Geometry check sheet. Reference: drawing and pictorial views, mm from the part's lowest x, y, z. A direction names the side the tool comes from. Give positions to 0.01 mm unless a question says otherwise; leave off trailing zeros. Order: outer loops, then holes, each group sorted by start corner. A loop starts at its lowest first (then second) coordinate and runs counter-clockwise, first axis right, second up.
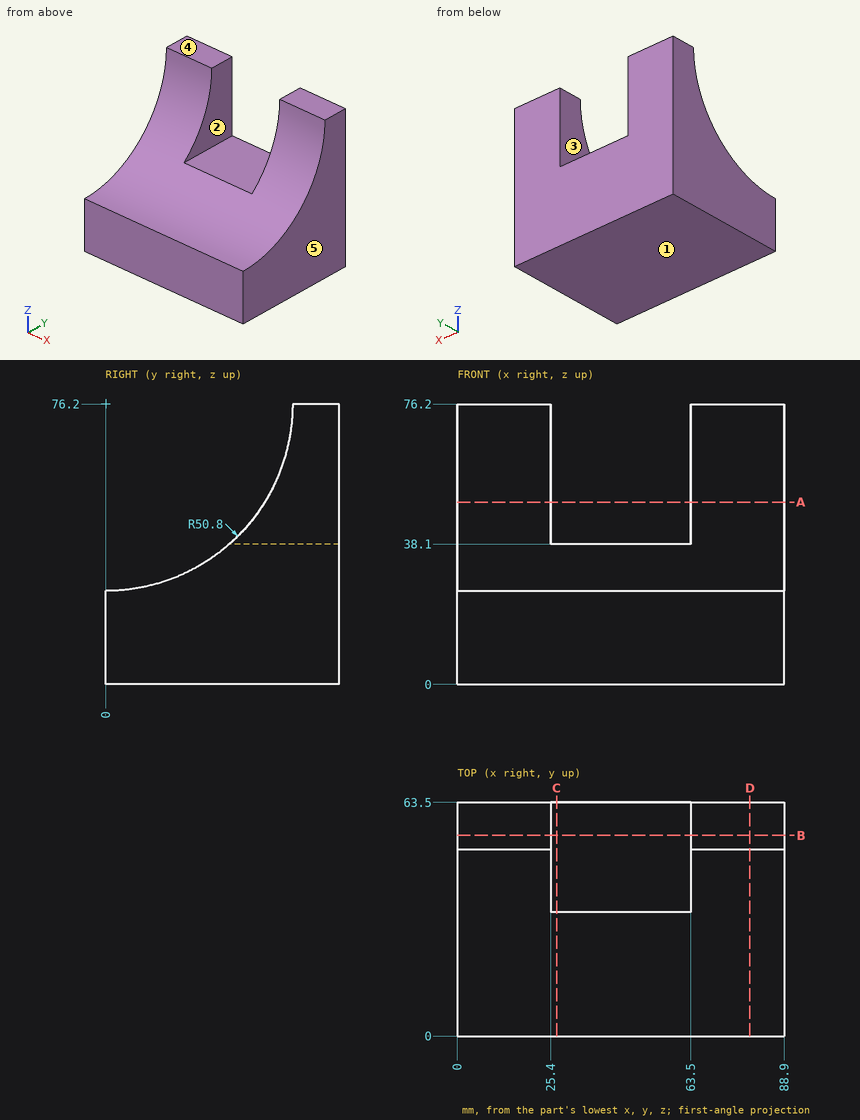
(1) Set-up check for the marked faces 1 and 2: record each of +Z, -Z, +X, -X, +Y, -Y from which the full face is reachable in a straight line by a thin tool's end or side.
Response values:
face 1: -Z, +X, -X, +Y, -Y
face 2: +Z, +Y, -Y
(2) Cross-section at C-C on x = 27. Enter the section's corners in (y, z).
Response values:
outline: (0, 0) - (63.5, 0) - (63.5, 38.1) - (33.6, 38.1) arc R50.8 cw to (0, 25.4) - close
(3) Cross-section at D-D on x = 79.5. Enter the section's corners in (y, z).
Response values:
outline: (0, 0) - (63.5, 0) - (63.5, 76.2) - (50.8, 76.2) arc R50.8 cw to (0, 25.4) - close
(4) Release check for a two-part mould opening along X. For the marked faces 3, 4 and 5 record: released by +X, released by -X, zero draft, split by the parting line, or undercut.
Response values:
face 3: undercut
face 4: zero draft
face 5: released by +X
(5) Cross-section at B-B on y = 54.5. Enter the section's corners in (x, z).
Response values:
outline: (0, 0) - (88.9, 0) - (88.9, 76.2) - (63.5, 76.2) - (63.5, 38.1) - (25.4, 38.1) - (25.4, 76.2) - (0, 76.2) - close
(6) Material ranges on L1, parallel to X at y = 35, z = 39; L2, parallel to Z at x = 29.5, y = 50.5; L3, parallel to Z at x = 33, y = 23, recorded low to high.
Response values:
L1: x = 0 to 25.4, 63.5 to 88.9
L2: z = 0 to 38.1
L3: z = 0 to 30.9
(7) Cross-section at A-A on z = 49.5. Enter the section's corners in (x, y), then the cut area to 3 significant figures.
Response values:
outline: (0, 43.22) - (25.4, 43.22) - (25.4, 63.5) - (0, 63.5) - close; (63.5, 43.22) - (88.9, 43.22) - (88.9, 63.5) - (63.5, 63.5) - close
area: 1,030 mm2
(8) Gauge pin test, flat end, axial feed: pin 1 Ø2 at (x, y) = (26.5, 17) entering from +Z. Record the tip position at first contact, or that the pin passes through.
Response values:
pin 1: stops at z = 28.7
